from build123d import *

# Parameters (mm, degrees)
ESBO_O1_W                = 100
ESBO_O1_H                = 95
RESSALTO_EXTRUS_O1_DEPTH = 1.5
ESBO_O3_W                = 3
ESBO_O3_H                = 32
RESSALTO_EXTRUS_O2_DEPTH = 3
ESBO_O2_R                = 1.5
ESBO_O2_W                = 40
ESBO_O2_H                = 3
CORTE_EXTRUS_O1_DEPTH    = 4
CUT_EXTRUDE7_DEPTH       = 2.5
CUT_EXTRUDE7_DEPTH_BACK  = 2.5
CUT_EXTRUDE5_DEPTH       = 2.5
CUT_EXTRUDE5_DEPTH_BACK  = 2.5
SKETCH7_W                = 13.5
SKETCH7_H                = 9.5
CUT_EXTRUDE6_DEPTH       = 2.5
CUT_EXTRUDE6_DEPTH_BACK  = 2.5
FILLET2_R                = 5


with BuildPart() as part:
    # Esboço1 → Ressalto-extrusão1 (new body, symmetric)
    with BuildSketch(Plane.XY):
        Rectangle(ESBO_O1_W, ESBO_O1_H)
    extrude(amount=RESSALTO_EXTRUS_O1_DEPTH, both=True)

    # Esboço3 → Ressalto-extrusão2 (add, through all)
    with BuildSketch(Plane.XY.offset(1.5)):
        with Locations((-51.5, 31.5)):
            Rectangle(ESBO_O3_W, ESBO_O3_H)
        with Locations((-51.5, -31.5)):
            Rectangle(ESBO_O3_W, ESBO_O3_H)
        with Locations((51.5, -31.5)):
            Rectangle(ESBO_O3_W, ESBO_O3_H)
        with Locations((51.5, 31.5)):
            Rectangle(ESBO_O3_W, ESBO_O3_H)
    extrude(amount=-RESSALTO_EXTRUS_O2_DEPTH)

    # Esboço2 → Corte-extrusão1 (cut, through all)
    with BuildSketch(Plane.XY.offset(1.5)):
        with Locations((-33, -1)):
            Circle(ESBO_O2_R)
        with Locations((33, -1)):
            Circle(ESBO_O2_R)
        with Locations((0, -46)):
            Rectangle(ESBO_O2_W, ESBO_O2_H)
        with Locations((0, -1)):
            Rectangle(ESBO_O2_W, ESBO_O2_H)
    extrude(amount=-CORTE_EXTRUS_O1_DEPTH, mode=Mode.SUBTRACT)

    # Sketch9 → Cut-Extrude7 (cut, two sides)
    with BuildSketch(Plane.XY) as cut_extrude7_sk:
        with BuildLine():
            Line((-1.5, -44.5), (1.5, -44.5))
            Line((1.5, -44.5), (1.5, -40.5))
            Line((1.5, -40.5), (2.85, -40.5))
            Line((2.85, -40.5), (2.85, -38.23))
            Line((2.85, -38.23), (1.5, -38.23))
            Line((1.5, -38.23), (1.5, -33.5))
            ThreePointArc((1.5, -33.5), (1.207106781, -32.792893219), (0.5, -32.5))
            Line((0.5, -32.5), (-0.5, -32.5))
            ThreePointArc((-0.5, -32.5), (-1.207106781, -32.792893219), (-1.5, -33.5))
            Line((-1.5, -33.5), (-1.5, -38.23))
            Line((-1.5, -38.23), (-2.85, -38.23))
            Line((-2.85, -38.23), (-2.85, -40.5))
            Line((-2.85, -40.5), (-1.5, -40.5))
            Line((-1.5, -40.5), (-1.5, -44.5))
        make_face()
    extrude(amount=CUT_EXTRUDE7_DEPTH, mode=Mode.SUBTRACT)
    extrude(cut_extrude7_sk.sketch, amount=-CUT_EXTRUDE7_DEPTH_BACK, mode=Mode.SUBTRACT)

    # Sketch6 → Cut-Extrude5 (cut, two sides)
    with BuildSketch(Plane.XY) as cut_extrude5_sk:
        with BuildLine():
            Line((-6, 44.5), (6, 44.5))
            ThreePointArc((6, 44.5), (7.414213562, 43.914213562), (8, 42.5))
            Line((8, 42.5), (8, 41))
            ThreePointArc((8, 41), (8.000003519, 40.99675088), (8.000014076, 40.993501776))
            ThreePointArc((8.000014076, 40.993501776), (8.25094791, 40.562114644), (8.750009384, 40.562655149))
            Line((8.750009384, 40.562655149), (9.75, 41.14))
            Line((9.75, 41.14), (12.469319768, 39.57))
            Line((12.469319768, 39.57), (12.469319768, 36.43))
            Line((12.469319768, 36.43), (9.75, 34.86))
            Line((9.75, 34.86), (8.750009384, 35.437344851))
            ThreePointArc((8.750009384, 35.437344851), (8.25094791, 35.437885356), (8.000014076, 35.006498224))
            ThreePointArc((8.000014076, 35.006498224), (8.000003519, 35.00324912), (8, 35))
            Line((8, 35), (8, 33.5))
            ThreePointArc((8, 33.5), (7.414213562, 32.085786438), (6, 31.5))
            Line((6, 31.5), (-6, 31.5))
            ThreePointArc((-6, 31.5), (-7.414213562, 32.085786438), (-8, 33.5))
            Line((-8, 33.5), (-8, 35))
            ThreePointArc((-8, 35), (-8.000003519, 35.00324912), (-8.000014076, 35.006498224))
            ThreePointArc((-8.000014076, 35.006498224), (-8.25094791, 35.437885356), (-8.750009384, 35.437344851))
            Line((-8.750009384, 35.437344851), (-9.75, 34.86))
            Line((-9.75, 34.86), (-12.469319768, 36.43))
            Line((-12.469319768, 36.43), (-12.469319768, 39.57))
            Line((-12.469319768, 39.57), (-9.75, 41.14))
            Line((-9.75, 41.14), (-8.750009384, 40.562655149))
            ThreePointArc((-8.750009384, 40.562655149), (-8.25094791, 40.562114644), (-8.000014076, 40.993501776))
            ThreePointArc((-8.000014076, 40.993501776), (-8.000003519, 40.99675088), (-8, 41))
            Line((-8, 41), (-8, 42.5))
            ThreePointArc((-8, 42.5), (-7.414213562, 43.914213562), (-6, 44.5))
        make_face()
    extrude(amount=CUT_EXTRUDE5_DEPTH, mode=Mode.SUBTRACT)
    extrude(cut_extrude5_sk.sketch, amount=-CUT_EXTRUDE5_DEPTH_BACK, mode=Mode.SUBTRACT)

    # Sketch7 → Cut-Extrude6 (cut, two sides)
    with BuildSketch(Plane.XY) as cut_extrude6_sk:
        with Locations((-33, 32.75)):
            Rectangle(SKETCH7_W, SKETCH7_H)
        with Locations((33, 32.75)):
            Rectangle(SKETCH7_W, SKETCH7_H)
    extrude(amount=CUT_EXTRUDE6_DEPTH, mode=Mode.SUBTRACT)
    extrude(cut_extrude6_sk.sketch, amount=-CUT_EXTRUDE6_DEPTH_BACK, mode=Mode.SUBTRACT)

    # Fillet2
    fillet2_edges = [part.edges().sort_by_distance(p)[0] for p in [
        (-53, 47.5, 0),
        (53, 47.5, 0),
    ]]
    fillet(fillet2_edges, radius=FILLET2_R)


solid = part.part
CAD build for the part. Positions are in the model's coordinates, mm. A direction names the side the tool comes from. Coordinates: 2 decimals unless noted, no trailing zeros. Write each loop counter-clockwise with the first axis right and the second up, starting at its lowest first coordinate (ties: lowest second). Pieces come first, ordered by that corner, then holes. Notation, with made-up numbers: (12, 68.25) - (62, 68.25) arc R17 cw to (62, 80.25) - close; hole circle Ø6 at (-30.5, 0.25). An arc over 180 degrees is marked (long way). Use a Markdown table: item, result. Add a question column.
Item 1: Band-saw the part on B-B, the plane y = -1. Give the cut face in (x, z).
Item 2: Flat gauge pins, fed straight in: pin 1 (1.1 mm diameter, centred on x = -2, z = -0.5, fed in from -Y); pin 2 (1.5 mm diameter, centred on y = -1, z = 0.5, fed in from -X); pin 3 (2.5 mm diameter, centred on x = 33, y = -1, fed in from -Z). Where does each tip first touch, or does it go through?
Item 3: 3-axis set-ups, long thin cutter, end or side, ignore diameter. For faces 1 (the face through (2.85, -39, 0)), 2 (the face through (-53, -32, 0)): which of +Z, -Z, +X, -X, +Y, -Y reach the whole face in a straight line?
Item 4: Drill centre lines: L1, parallel to Y at x = 3.5, z = 0.5; L2, parallel to Y at x = -8.5, z = -0.6; L3, parallel to X at y = 33.5, z = -1.1. Where is each one in solid material? Low to high. Write a range as from..to.
Item 5: Band-saw the part on A-A, the plane x = -33. Give the cut face in (y, z).
Item 6: Band-saw the part on D-D, the plane y = -13.5. Give the cut face in (x, z), and give its area (3 significant figures).
Item 7: Mould opens along Y. For faces 3 (the face through (11.129, 35.656, -0.021)), 4 (the face through (20, -46, 0)), 5 (the face through (-11, -44.5, 0)), 6 (the face through (0, 31.5, 0)) say: pulls with the +Y half, pulls with the -Y half, needs draft (parallel to the pull), parting line crosses it, or undercut.
Item 8: Band-saw the part on C-C, the plane z = -0.7. Give the number of separate pieces and of enclosed holes in the cut face, and give its area (3 significant figures).
Numbers:
| question | item | result |
|---|---|---|
| 1 | outline | (-50, -1.5) - (-34.5, -1.5) - (-34.5, 1.5) - (-50, 1.5) - close; (-31.5, -1.5) - (-20, -1.5) - (-20, 1.5) - (-31.5, 1.5) - close; (20, -1.5) - (31.5, -1.5) - (31.5, 1.5) - (20, 1.5) - close; (34.5, -1.5) - (50, -1.5) - (50, 1.5) - (34.5, 1.5) - close |
| 2 | pin 1 | y = -44.5 |
| 2 | pin 2 | x = -50 |
| 2 | pin 3 | through |
| 3 | face 1 | +Z, -Z |
| 3 | face 2 | +Z, -Z, -X, +Y, -Y |
| 4 | L1 | -44.5..-2.5, 0.5..31.5, 44.5..47.5 |
| 4 | L2 | -44.5..-2.5, 0.5..35.5, 40.5..47.5 |
| 4 | L3 | -53..-39.75, -26.25..-8, 8..26.25, 39.75..53 |
| 5 | outline | (-47.5, -1.5) - (-2.5, -1.5) - (-2.5, 1.5) - (-47.5, 1.5) - close; (0.5, -1.5) - (28, -1.5) - (28, 1.5) - (0.5, 1.5) - close; (37.5, -1.5) - (47.5, -1.5) - (47.5, 1.5) - (37.5, 1.5) - close |
| 6 | outline | (-50, -1.5) - (50, -1.5) - (50, 1.5) - (-50, 1.5) - close |
| 6 | area | 300 mm2 |
| 7 | face 3 | undercut |
| 7 | face 4 | needs draft |
| 7 | face 5 | pulls with the -Y half |
| 7 | face 6 | undercut |
| 8 | separate pieces | 1 |
| 8 | enclosed holes | 6 |
| 8 | area | 9,070 mm2 |
